from build123d import *

# Parameters (mm, degrees)
SKETCH_1_W      = 60
SKETCH_1_H      = 63.5
SKETCH_1_R      = 12
SKETCH_1_R_2    = 4
EXTRUDE_1_DEPTH = 10
CHAMFER_1_SIZE  = 0.25
SKETCH_2_W      = 60
SKETCH_2_H      = 5
EXTRUDE_2_DEPTH = 60
MM_START        = -31.75
MM_1_DEPTH      = 5


# Read off the part's stored shape, not the designer's step: 大小mm 暗销槽口1
with BuildPart() as part:
    # 草图1 → 凸台-拉伸1 (new body)
    with BuildSketch(Plane.XY):
        Rectangle(SKETCH_1_W, SKETCH_1_H)
        Circle(SKETCH_1_R, mode=Mode.SUBTRACT)
        with Locations((20, 0)):
            Circle(SKETCH_1_R_2, mode=Mode.SUBTRACT)
        with Locations(Location((-20, 0, 0), (0, 0, 180))):
            Circle(SKETCH_1_R_2, mode=Mode.SUBTRACT)
    extrude(amount=EXTRUDE_1_DEPTH)

    # 倒角1
    chamfer_1_edges = [part.edges().sort_by_distance(p)[0] for p in [
        (16, 0, 0),
        (-16, 0, 0),
    ]]
    chamfer(chamfer_1_edges, length=CHAMFER_1_SIZE)

    # 草图2 → 凸台-拉伸2 (add)
    with BuildSketch(Plane.XY.offset(10)):
        with Locations((0, -29.25)):
            Rectangle(SKETCH_2_W, SKETCH_2_H)
    extrude(amount=EXTRUDE_2_DEPTH)

    # 大小mm 暗销槽口1 outline → 大小mm 暗销槽口1 (cut)
    with BuildSketch(Plane(origin=(0, 0, 0), x_dir=(1, 0, 0), z_dir=(0, 1, 0)).offset(MM_START)):
        with BuildLine():
            ThreePointArc((23.909259259, -32.749042146), (25.459259259, -34.299042146), (27.009259259, -32.749042146))
            Line((27.009259259, -32.749042146), (27.009259259, -22.749042146))
            ThreePointArc((27.009259259, -22.749042146), (25.459259259, -21.199042146), (23.909259259, -22.749042146))
            Line((23.909259259, -22.749042146), (23.909259259, -32.749042146))
        make_face()
        with BuildLine():
            Line((27.009259259, -67.557471264), (27.009259259, -57.557471264))
            ThreePointArc((27.009259259, -57.557471264), (25.459259259, -56.007471264), (23.909259259, -57.557471264))
            Line((23.909259259, -57.557471264), (23.909259259, -67.557471264))
            ThreePointArc((23.909259259, -67.557471264), (25.459259259, -69.107471264), (27.009259259, -67.557471264))
        make_face()
        with BuildLine():
            Line((-23.909259259, -67.557471264), (-23.909259259, -57.557471264))
            ThreePointArc((-23.909259259, -57.557471264), (-25.459259259, -56.007471264), (-27.009259259, -57.557471264))
            Line((-27.009259259, -57.557471264), (-27.009259259, -67.557471264))
            ThreePointArc((-27.009259259, -67.557471264), (-25.459259259, -69.107471264), (-23.909259259, -67.557471264))
        make_face()
        with BuildLine():
            Line((-23.909259259, -32.749042146), (-23.909259259, -22.749042146))
            ThreePointArc((-23.909259259, -22.749042146), (-25.459259259, -21.199042146), (-27.009259259, -22.749042146))
            Line((-27.009259259, -22.749042146), (-27.009259259, -32.749042146))
            ThreePointArc((-27.009259259, -32.749042146), (-25.459259259, -34.299042146), (-23.909259259, -32.749042146))
        make_face()
    extrude(amount=MM_1_DEPTH, mode=Mode.SUBTRACT)


solid = part.part
CAD build for the part. Positions are in the model's coordinates, mm. A direction names the side the tool comes from. Coordinates: 2 decimals unless noted, no trailing zeros. Write each loop counter-clockwise with the first axis right and the second up, starting at its lowest first coordinate (ties: lowest second). Pieces come first, ordered by that corner, then holes. Notation, with made-up numbers: (40, 60.5) - (60, 60.5) arc R22 cw to (60, 66.5) - close; hole circle Ø5 at (77, 20.25). An arc over 180 degrees is marked (long way). Use a Markdown table: item, result. Add a question column.
Item 1: Mould opens along Y. For faces 4 (the face through (0, 31.75, 5)), 5 (the face through (16.8, -2.4, 5.1)), 6 (the face through (0, -31.75, 35)) say: pulls with the +Y half, pulls with the -Y half, needs draft (parallel to the pull), parting line crosses it, or undercut.
Item 2: 3-axis set-ups, long thin cutter, end or side, ignore diameter. For faces 1 (the face through (27.009, -29, 28)), 2 (the face through (0, 16, 10)), 3 (the face through (0, -29, 70)): which of +Z, -Z, +X, -X, +Y, -Y reach the whole face in a straight line?
Item 3: Drill centre lines: L1, parallel to Y at x = 0, z = 2; L2, parallel to Y at x = -20, z = 6.25; L3, parallel to Z at x = -9, y = -19.5. Where is each one in solid material? Low to high. Write a range as from..to.
Item 4: Band-saw the part on B-B, the plane z = 64.5. Give the cut face in (x, y).
Item 5: Band-saw the part on D-D, the plane x = 0. Give the cut face in (y, z), and give its area (3 significant figures).
Item 6: Band-saw the part on C-C, the plane y = 0. Give the cut face in (x, z).
Item 7: Flat gauge pins, fed straight in: pin 1 (6 mm diameter, centred on x = 21, y = -1.5, fed in from -Z); pin 2 (18 mm diameter, centred on x = 9.5, z = 28, fed in from +Y). Where does each tip first touch, or does it go through?
Item 8: Band-saw the part on A-A, the plane x = -20. Give the cut face in (y, z), and give its area (3 significant figures).
Numbers:
| question | item | result |
|---|---|---|
| 1 | face 4 | pulls with the +Y half |
| 1 | face 5 | undercut |
| 1 | face 6 | pulls with the -Y half |
| 2 | face 1 | +Y, -Y |
| 2 | face 2 | +Z, +X, -X, +Y |
| 2 | face 3 | +Z, +X, -X, +Y, -Y |
| 3 | L1 | -31.75..-12, 12..31.75 |
| 3 | L2 | -31.75..-4, 4..31.75 |
| 3 | L3 | 0..10 |
| 4 | outline | (-30, -31.75) - (-27.01, -31.75) - (-27.01, -26.75) - (-30, -26.75) - close; (-23.91, -31.75) - (23.91, -31.75) - (23.91, -26.75) - (-23.91, -26.75) - close; (27.01, -31.75) - (30, -31.75) - (30, -26.75) - (27.01, -26.75) - close |
| 5 | outline | (-31.75, 0) - (-12, 0) - (-12, 10) - (-26.75, 10) - (-26.75, 70) - (-31.75, 70) - close; (12, 0) - (31.75, 0) - (31.75, 10) - (12, 10) - close |
| 5 | area | 695 mm2 |
| 6 | outline | (-30, 0) - (-24.25, 0) - (-24, 0.25) - (-24, 10) - (-30, 10) - close; (-16, 0.25) - (-15.75, 0) - (-12, 0) - (-12, 10) - (-16, 10) - close; (12, 0) - (15.75, 0) - (16, 0.25) - (16, 10) - (12, 10) - close; (24, 0.25) - (24.25, 0) - (30, 0) - (30, 10) - (24, 10) - close |
| 7 | pin 1 | z = 0 |
| 7 | pin 2 | y = -26.75 |
| 8 | outline | (-31.75, 0) - (-4.25, 0) - (-4, 0.25) - (-4, 10) - (-26.75, 10) - (-26.75, 70) - (-31.75, 70) - close; (4, 0.25) - (4.25, 0) - (31.75, 0) - (31.75, 10) - (4, 10) - close |
| 8 | area | 855 mm2 |
